Here's how the part is built. I have some questions about the finished solid (model axes, mm). A direction names the side the tool comes from. Coordinates: 2 decimals unless noted, no trailing zeros. Write each loop counter-clockwise with the first axis right and the second up, starting at its lowest first coordinate (ties: lowest second). Pieces come first, ordered by that corner, then holes.
(1) Please list where these lines run through material, in increasing order: probe 1 along Y at (x, z) = (101.5, 0.35); probe 2 along Y at (x, z) = (163.5, 2.1); probe 3 along Y at (x, z) = (43, 0.95).
(2) Imagine slicing it at A-A, the plane x = 168.5. List the corners of the cut face in (y, z) for me, plus the area to 3 significant figures.
(3) Imagine slicing it at B-B, the plane x = 129. List the corners of the cut face in (y, z) for me.
(4) For pin 1 Ø3 at (x, z) = (71, 1.5) entering from +Y; pin 2 Ø1.5 at (x, z) = (99.5, 5.5) entering from -Y; pin 3 Ø3 at (x, y) = (51.39, 58.68) entering from +Z; pin 4 Ø3 at (y, z) = (11, 4) entering from -X, each with a flat end and sliding along its axis, tell me the tip position at first contact or that it passes through.
(5) Which directions (+Z, -Z, +X, -X, +Y, -Y) give clear straight access to the entire face, cutting with the end or side of a thin tool? Please do faces 1 (the flat face through (121.391, 166, 3)), 2 (the flat face through (114, 169.181, 3)), 3 (the flat face through (98, 108, 0)), 4 (the flat face through (39, 13.681, 3)), 5 (the flat face through (113, 103.681, 3)).
(6) Imagine slicing it at C-C, the plane z = 4.65. State how many separate pieces and enclosed holes the cut face has, plus the area to 3 significant figures.
```python
from build123d import *

# Parameters (mm, degrees)
MODEL_R             = 2
BOSS_EXTRUDE1_DEPTH = 6
SKETCH2_W           = 6
SKETCH2_H           = 150
BOSS_EXTRUDE2_DEPTH = 1


with BuildPart() as part:
    # Model → Boss-Extrude1 (new body)
    with BuildSketch(Plane.XY):
        with BuildLine():
            Line((31.391248016, 13.680569099), (46.391248016, 13.680569099))
            Line((46.391248016, 13.680569099), (46.391248016, 8.180569099))
            Line((46.391248016, 8.180569099), (61.391248016, 8.180569099))
            Line((61.391248016, 8.180569099), (61.391248016, 13.680569099))
            Line((61.391248016, 13.680569099), (76.391248016, 13.680569099))
            Line((76.391248016, 13.680569099), (76.391248016, 8.180569099))
            Line((76.391248016, 8.180569099), (91.391248016, 8.180569099))
            Line((91.391248016, 8.180569099), (91.391248016, 13.680569099))
            Line((91.391248016, 13.680569099), (106.391248016, 13.680569099))
            Line((106.391248016, 13.680569099), (106.391248016, 8.180569099))
            Line((106.391248016, 8.180569099), (121.391248016, 8.180569099))
            Line((121.391248016, 8.180569099), (121.391248016, 13.680569099))
            Line((121.391248016, 13.680569099), (136.391248016, 13.680569099))
            Line((136.391248016, 13.680569099), (136.391248016, 8.180569099))
            Line((136.391248016, 8.180569099), (151.391248016, 8.180569099))
            Line((151.391248016, 8.180569099), (151.391248016, 13.680569099))
            Line((151.391248016, 13.680569099), (166.391248016, 13.680569099))
            Line((166.391248016, 13.680569099), (166.391248016, 8.180569099))
            Line((166.391248016, 8.180569099), (181.391248016, 8.180569099))
            Line((181.391248016, 8.180569099), (181.391248016, 73.680569099))
            Line((181.391248016, 73.680569099), (46.391248016, 73.680569099))
            ThreePointArc((46.391248016, 73.680569099), (31.391248016, 88.680569099), (46.391248016, 103.680569099))
            Line((46.391248016, 103.680569099), (181.391248016, 103.680569099))
            Line((181.391248016, 103.680569099), (181.391248016, 169.180569099))
            Line((181.391248016, 169.180569099), (166.391248016, 169.180569099))
            Line((166.391248016, 169.180569099), (166.391248016, 163.680569099))
            Line((166.391248016, 163.680569099), (151.391248016, 163.680569099))
            Line((151.391248016, 163.680569099), (151.391248016, 169.180569099))
            Line((151.391248016, 169.180569099), (136.391248016, 169.180569099))
            Line((136.391248016, 169.180569099), (136.391248016, 163.680569099))
            Line((136.391248016, 163.680569099), (121.391248016, 163.680569099))
            Line((121.391248016, 163.680569099), (121.391248016, 169.180569099))
            Line((121.391248016, 169.180569099), (106.391248016, 169.180569099))
            Line((106.391248016, 169.180569099), (106.391248016, 163.680569099))
            Line((106.391248016, 163.680569099), (91.391248016, 163.680569099))
            Line((91.391248016, 163.680569099), (91.391248016, 169.180569099))
            Line((91.391248016, 169.180569099), (76.391248016, 169.180569099))
            Line((76.391248016, 169.180569099), (76.391248016, 163.680569099))
            Line((76.391248016, 163.680569099), (61.391248016, 163.680569099))
            Line((61.391248016, 163.680569099), (61.391248016, 169.180569099))
            Line((61.391248016, 169.180569099), (46.391248016, 169.180569099))
            Line((46.391248016, 169.180569099), (46.391248016, 163.680569099))
            Line((46.391248016, 163.680569099), (31.391248016, 163.680569099))
            Line((31.391248016, 163.680569099), (31.391248016, 169.180569099))
            Line((31.391248016, 169.180569099), (18.391248016, 169.180569099))
            Line((18.391248016, 169.180569099), (18.391248016, 8.180569099))
            Line((18.391248016, 8.180569099), (31.391248016, 8.180569099))
            Line((31.391248016, 8.180569099), (31.391248016, 13.680569099))
        make_face()
        with Locations((51.391248016, 58.680569099)):
            Circle(MODEL_R, mode=Mode.SUBTRACT)
        with Locations((101.391248016, 58.680569099)):
            Circle(MODEL_R, mode=Mode.SUBTRACT)
        with Locations((151.391248016, 58.680569099)):
            Circle(MODEL_R, mode=Mode.SUBTRACT)
        with Locations((42.423326125, 38.680569099)):
            Circle(MODEL_R, mode=Mode.SUBTRACT)
        with Locations((156.391248016, 38.680569099)):
            Circle(MODEL_R, mode=Mode.SUBTRACT)
        with Locations((51.391248016, 118.680569099)):
            Circle(MODEL_R, mode=Mode.SUBTRACT)
        with Locations((101.391248016, 118.680569099)):
            Circle(MODEL_R, mode=Mode.SUBTRACT)
        with Locations((151.391248016, 118.680569099)):
            Circle(MODEL_R, mode=Mode.SUBTRACT)
        with Locations((42.423326125, 138.680569099)):
            Circle(MODEL_R, mode=Mode.SUBTRACT)
        with Locations((156.391248016, 138.680569099)):
            Circle(MODEL_R, mode=Mode.SUBTRACT)
    extrude(amount=BOSS_EXTRUDE1_DEPTH)

    # Sketch2 → Boss-Extrude2 (add)
    with BuildSketch(Plane.ZY.offset(-18.391248016)):
        with Locations((3, 88.680569099)):
            Rectangle(SKETCH2_W, SKETCH2_H)
    extrude(amount=BOSS_EXTRUDE2_DEPTH)


solid = part.part
```
Recorded:
1. probe 1: y = 13.68 to 56.68, 60.68 to 73.68, 103.68 to 116.68, 120.68 to 163.68
1. probe 2: y = 13.68 to 73.68, 103.68 to 163.68
1. probe 3: y = 13.68 to 36.77, 40.6 to 74.07, 103.29 to 136.77, 140.6 to 163.68
2. outline: (8.18, 0) - (73.68, 0) - (73.68, 6) - (8.18, 6) - close; (103.68, 0) - (169.18, 0) - (169.18, 6) - (103.68, 6) - close
2. area: 786 mm2
3. outline: (13.68, 0) - (73.68, 0) - (73.68, 6) - (13.68, 6) - close; (103.68, 0) - (163.68, 0) - (163.68, 6) - (103.68, 6) - close
4. pin 1: stops at y = 163.68
4. pin 2: stops at y = 13.68
4. pin 3: passes through
4. pin 4: stops at x = 18.39
5. face 1: +Z, -Z, +Y
5. face 2: +Z, -Z, +X, -X, +Y
5. face 3: -Z, +X, -X, +Y, -Y
5. face 4: +Z, -Z, -Y
5. face 5: +Z, -Z, +X
6. separate pieces: 1
6. enclosed holes: 10
6. area: 21,000 mm2
